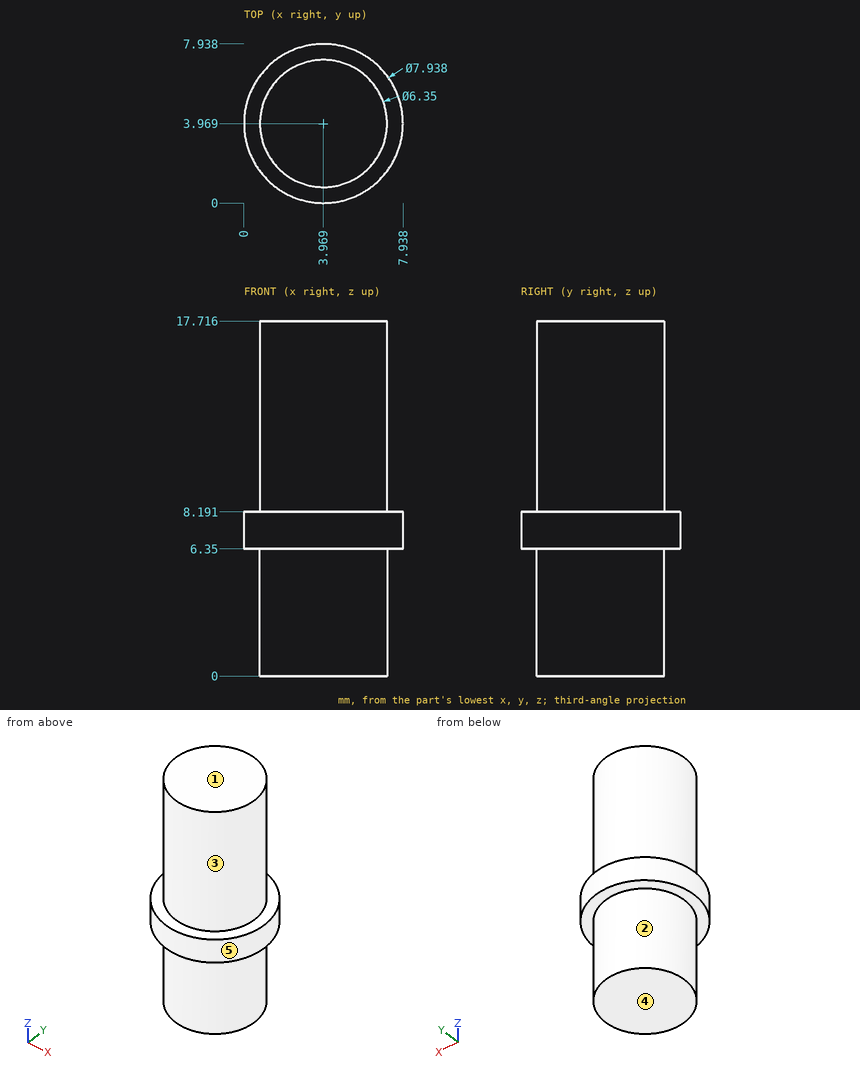
Verification items for this drawing (mm, ordinates from the low corner). A direction names the side the tool comes from. Coordinates: 2 decimals unless noted, no trailing zeros. Answer in a Markdown table with one row per item. Add a question column.
1. Depth check by flat-ended pin: P1, Ø2, axis at y = 4, z = 14, coming from the -X side; P2, Ø1, axis at x = 3, z = 10.5, coming from the +Y side; P3, Ø1, axis at y = 6.5, z = 11.5, coming from the -X side. Enter the tip coordinate at first touch or a pass-through.
2. Material ranges on probe 1 along Z at (x, y) = (1, 2.25); probe 2 along X at (y, z) = (5.5, 9.5); probe 3 along Y at (x, z) = (2.5, 6) (1 decimal), recorded low to high. Write a range as [from, to].
3. Access from +Z, -Z, +X, -X, +Y, -Y to the whole of each face (thin tool, end or side, straight path). Record for the marked faces 1, 2 and 3.
4. Draft check along Y on the marked faces 4 and 5. Enter one of: +Y half, -Y half, draft (parallel to the pull), parting line (faces both ways), or undercut.
Derived:
| question | item | result |
|---|---|---|
| 1 | P1 | stops at x = 0.79 |
| 1 | P2 | stops at y = 7.11 |
| 1 | P3 | stops at x = 1.53 |
| 2 | probe 1 | z = [6.35, 8.19] |
| 2 | probe 2 | x = [1.19, 6.75] |
| 2 | probe 3 | y = [1.2, 6.8] |
| 3 | face 1 | +Z, +X, -X, +Y, -Y |
| 3 | face 2 | -Z |
| 3 | face 3 | +Z |
| 4 | face 4 | draft |
| 4 | face 5 | parting line |
